The listing builds one solid part. Answer for the finished solid, in the listing's coordinates (mm). Coordinates: 2 decimals unless noted, no trailing zeros. Order: outer loops, then holes, each group sorted by start corner. A loop starts at its lowest first (then second) coordinate and runs counter-clockwise, first axis right, second up.
```python
from build123d import *

# Parameters (mm, degrees)
F0_W     = 60
F0_H     = 60
F1_DEPTH = 4
F2_D     = 5
F3_R     = 2.5


with BuildPart() as f1:
    # F0 (on Front) → F1 (new body)
    with BuildSketch(Plane.XZ):
        Rectangle(F0_W, F0_H)
    extrude(amount=F1_DEPTH)

    # F2 (through all)
    with Locations(Plane(origin=(0, 0, 0), x_dir=(1, 0, 0), z_dir=(0, 1, 0))):
        with Locations((-20.3, -20.3), (20.3, -20.3), (20.3, 20.3), (-20.3, 20.3), (0, 20.3), (20.3, 0), (0, -20.3), (-20.3, 0)):
            Hole(F2_D / 2)

    # F3
    f3_edges = [f1.edges().sort_by_distance(p)[0] for p in [
        (30, -2, 30),
        (30, -2, -30),
        (-30, -2, -30),
        (-30, -2, 30),
    ]]
    fillet(f3_edges, radius=F3_R)


solid = f1.part
```
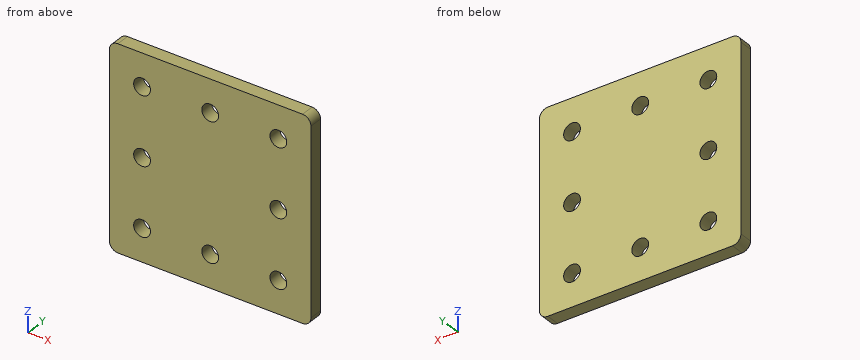
(1) Find section B-B (y = -0.9). Give the number of separate pieces and of enclosed holes in the cut face, and give its area (3 significant figures).
(2) Find section C-C (z = -20.3). Write down the section's boundary in (x, y), and give its area (3 significant figures).
(3) Consider line 1 (Z direction, x = 0, y = -1.9); line 2 (Z direction, x = -20.3, y = -2.3). Determine where each line is inside the solid, lowest interval first.
(4) Find section D-D (x = -20.3). Write down the section's boundary in (y, z).
(5) Find section A-A (x = 0). Write down the section's boundary in (y, z).
Findings below:
1. separate pieces: 1
1. enclosed holes: 8
1. area: 3,440 mm2
2. outline: (-30, -4) - (-22.8, -4) - (-22.8, 0) - (-30, 0) - close; (-17.8, -4) - (-2.5, -4) - (-2.5, 0) - (-17.8, 0) - close; (2.5, -4) - (17.8, -4) - (17.8, 0) - (2.5, 0) - close; (22.8, -4) - (30, -4) - (30, 0) - (22.8, 0) - close
2. area: 180 mm2
3. line 1: z = -30 to -22.8, -17.8 to 17.8, 22.8 to 30
3. line 2: z = -30 to -22.8, -17.8 to -2.5, 2.5 to 17.8, 22.8 to 30
4. outline: (-4, -30) - (0, -30) - (0, -22.8) - (-4, -22.8) - close; (-4, -17.8) - (0, -17.8) - (0, -2.5) - (-4, -2.5) - close; (-4, 2.5) - (0, 2.5) - (0, 17.8) - (-4, 17.8) - close; (-4, 22.8) - (0, 22.8) - (0, 30) - (-4, 30) - close
5. outline: (-4, -30) - (0, -30) - (0, -22.8) - (-4, -22.8) - close; (-4, -17.8) - (0, -17.8) - (0, 17.8) - (-4, 17.8) - close; (-4, 22.8) - (0, 22.8) - (0, 30) - (-4, 30) - close
